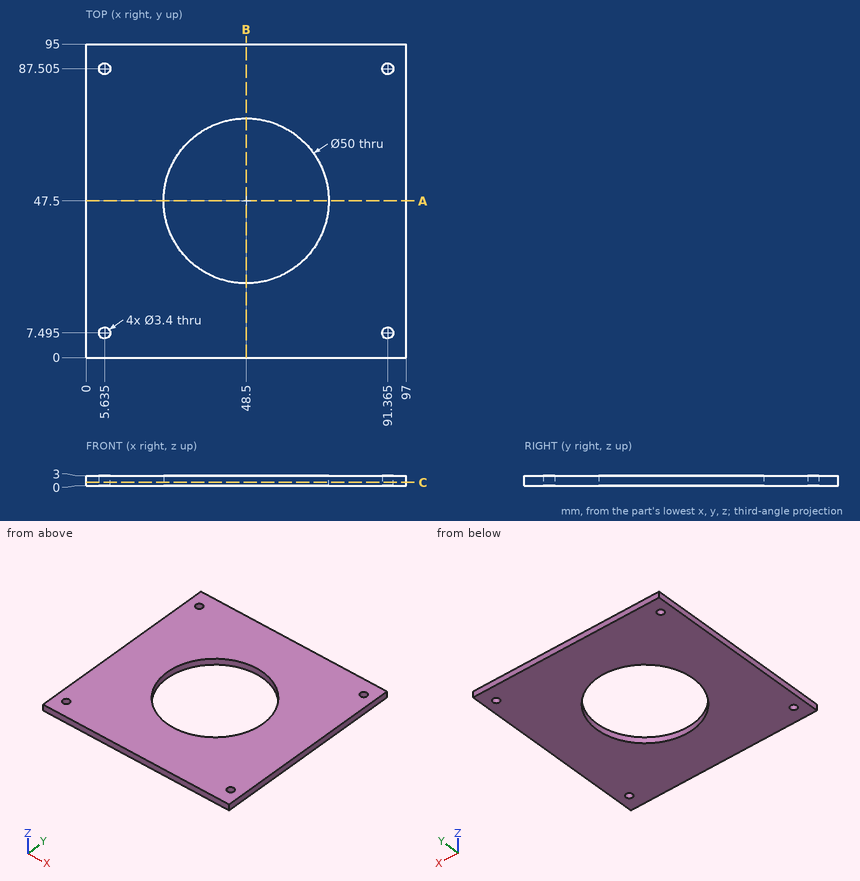
For this review, use the dimensioned drawing (mm, ordinates from the lowest corner) and the shaded views. Give positions to 0.01 mm unless a question says otherwise; leave off trailing zeros. Loops run counter-clockwise (first coordinate to the right, second up) from the corner with the lowest first, then second, coordinate; pieces in that order, holes last. Notation, with made-up numbers: (28, 68.25) - (42, 68.25) arc R24 cw to (42, 106.25) - close; hole circle Ø8 at (-16.75, -20.75). An arc over 180 degrees is marked (long way). Write each question's results on one line, items separated by ' | '.
(1) For line 1 along Y through (x, z) = (48.5, 1.2); line 2 along X through (y, z) = (88, 1); line 3 along X through (y, z) = (58, 1.9), list the stretches that pass through material, from the lowest coordinate up.
Conclusion:
line 1: 0 to 22.5, 72.5 to 95 | line 2: 0 to 4.01, 7.26 to 89.74, 92.99 to 97 | line 3: 0 to 25.81, 71.19 to 97
(2) Take a section at B-B (x = 48.5). Give the boundary of the cut face in (y, z).
Conclusion:
outline: (0, 0) - (22.5, 0) - (22.5, 3) - (0, 3) - close; (72.5, 0) - (95, 0) - (95, 3) - (72.5, 3) - close
(3) For pin 1 Ø1.5 at (x, z) = (48.5, 1) entering from -Y, flat-tipped, find the tip position at first contact; note if it passes through.
Conclusion:
pin 1: y = 0
(4) Take a section at A-A (y = 47.5). Give the boundary of the cut face in (x, z), then the cut area to 3 significant figures.
Conclusion:
outline: (0, 0) - (23.5, 0) - (23.5, 3) - (0, 3) - close; (73.5, 0) - (97, 0) - (97, 3) - (73.5, 3) - close | area: 141 mm^2
(5) Take a section at C-C (z = 0.95). Give the boundary of the cut face in (x, y) (3 decimals).
Conclusion:
outline: (0, 0) - (97, 0) - (97, 95) - (0, 95) - close; hole circle Ø3.4 at (5.635, 7.495); hole circle Ø3.4 at (5.635, 87.505); hole circle Ø50 at (48.5, 47.5); hole circle Ø3.4 at (91.365, 7.495); hole circle Ø3.4 at (91.365, 87.505)
